Part model, mm, in its own coordinate system. A direction names the side the tool comes from. Round coordinates to 2 decimals unless told otherwise and drop trailing zeros. Loops run counter-clockwise (first coordinate to the right, second up) from the corner with the lowest first, then second, coordinate; pieces in that order, holes last.
1) Probe line 1 (Y direction, x = -3.81, z = -8.5); line 2 (X direction, y = 5.5, z = -10.5); line 3 (Y direction, x = -0.75, z = -4). List the from-to ranges inside material, lowest first.
2) Band-saw the part on C-C, the plane x = -17.75. Write the cut outline in (y, z).
3) Band-saw the part on B-B, the plane y = 10. Write the cut outline in (x, z), then the cut area to 3 significant figures.
4) Drop flat-ended pins along their axis: P1, Ø4, axis at x = -3.5, y = 11, coming from the +Z side; P2, Ø2, axis at y = 4, z = -7, coming from the -X side; P3, Ø3, axis at y = 10.5, z = -4.5, coming from the +X side; P4, Ø4, axis at y = 8, z = -7, coming from the -X side. Give the stop position or say it passes through.
5) 3-axis set-ups, long thin cutter, end or side, ignore diameter. For faces 1 (the flat face through (-4, 6, -4.826)), 2 (the cylindrical face through (-6.474, 11.614, -8.082)): which of +Z, -Z, +X, -X, +Y, -Y reach the whole face in a straight line?
6) Mould opens along X. For faces 3 (the cylindrical face through (-4.05, 10.73, -8.08)), 4 (the flat face through (-7.62, 7, -8)), 5 (the flat face through (-4, 6, -11.43)) say: +X half, -X half, draft (parallel to the pull), parting line (faces both ways), or undercut.
7) Band-saw the part on D-D, the plane y = 12.25. Write the cut outline in (x, z).
8) Band-saw the part on A-A, the plane x = -3. Write the cut outline in (y, z).
Autodesk Inventor part; units mm, degrees
ref_plane "YZ Plane" through (0, 0, 0) normal (1, 0, 0) x (0, 1, 0)
ref_plane "XZ Plane" through (0, 0, 0) normal (0, 1, 0) x (-1, 0, 0)
ref_plane "XY Plane" through (0, 0, 0) normal (0, 0, 1) x (1, 0, 0)
sketch "Sketch1" plane through (0, 0, 0) normal (0, 1, 0) x (-1, 0, 0)
  line L0 (0, 0) -> (21.59, 0)
  line L1 (21.59, 0) -> (21.59, -22.86)
  line L2 (21.59, -22.86) -> (0, -22.86)
  line L3 (0, -22.86) -> (0, 0)
  line L4 (6.35, 0) -> (6.35, -22.86) construction
  circle A0 centre (8.382, -3.7846) radius 0.762
  circle A1 centre (8.382, -19.0754) radius 0.762
  line L5 (6.35, -3.7846) -> (7.62, -3.7846) construction
  line L6 (8.382, -3.0226) -> (8.382, 0) construction
  line L7 (7.62, -19.0754) -> (6.35, -19.0754) construction
  line L8 (8.382, -19.8374) -> (8.382, -22.86) construction
  line L9 (17.653, -10.287) -> (15.367, -10.287) construction
  line L10 (15.367, -10.287) -> (15.367, -12.573) construction
  line L11 (15.367, -12.573) -> (17.653, -12.573) construction
  line L12 (17.653, -12.573) -> (17.653, -10.287) construction
  line L13 (17.653, -11.43) -> (15.367, -11.43) construction
  line L14 (16.51, -10.287) -> (16.51, -12.573) construction
  line L15 (8.382, -19.0754) -> (8.382, -3.7846) construction
  point P0 (6.35, -11.43)
  dimension "d0" = 22.86
  dimension "d1" = 21.59
  dimension "d2" = 1.524
  dimension "d3" = 1.524
  dimension "d4" = 1.27
  dimension "d6" = 1.27
  dimension "d10" = 15.24
  dimension "d11" = 2.286
  dimension "d12" = 2.286
  dimension "d13" = 10.16
  dimension "d14" = 16.51
  dimension "d30" = 15.2908
  dimension "d31" = 3.0226
extrude "Extrusion1" add sketch "Sketch1" along normal blind 3.81
sketch "Sketch2" plane through (0, 3.81, 0) normal (0, 1, 0) x (1, 0, 0)
  line L0 (-21.59, 22.86) -> (-21.59, 0)
  line L1 (-21.59, 11.43) -> (0, 11.43) construction
  line L2 (0, 0) -> (0, 22.86)
  line L3 (0, 11.43) -> (-7.62, 11.43)
  line L4 (-7.62, 11.43) -> (-7.62, 4.826)
  line L5 (-7.62, 4.826) -> (0, 4.826)
  line L6 (0, 4.826) -> (0, 11.43)
  dimension "d17" = 6.604
  dimension "d18" = 7.62
extrude "Extrusion2" add sketch "Sketch2" along normal blind 8.89
fillet "Fillet1" radius 3.81 2 edges at (-7.62, 12.7, -8.128) (0, 12.7, -8.128)
sketch "Sketch3" plane through (-7.62, 3.81, -4.826) normal (0, 0, 1) x (1, 0, 0)
  arc A0 (7.62, 5.08) -> (0, 5.08) centre (3.81, 5.08) ccw
  circle A1 centre (3.81, 5.08) radius 1.8542
  point P0 (7.62, -3.81)
  dimension "d22" = 3.7084
extrude "Extrusion4" cut sketch "Sketch3" against normal through all
chamfer "Chamfer1" distance 1.27 angle 45 1 edges at (-7.62, 3.81, -8.128)
fillet "Fillet2" radius 1.27 4 edges at (-21.59, 1.905, 0) (0, 1.905, 0) (0, 1.905, -22.86) (-21.59, 1.905, -22.86)
equation "\"d3\" = d2"
equation "\"d6\" = d4"
equation "\"d31\" = -0.5 * d2 + 0.5 * d0 - 0.5 * d30"
properties part number "Mount for TMP007 Sensor"
Reported:
1. line 1: y = 0 to 7.04, 10.74 to 12.7
1. line 2: x = -7.62 to 0
1. line 3: y = 0 to 3.81
2. outline: (0, -22.86) - (3.81, -22.86) - (3.81, 0) - (0, 0) - close
3. outline: (-7.45, -11.43) - (-5.3, -11.43) - (-5.3, -4.83) - (-7.45, -4.83) - close; (-2.32, -11.43) - (-0.17, -11.43) - (-0.17, -4.83) - (-2.32, -4.83) - close
3. area: 28.5 mm2
4. P1: stops at z = -4.83
4. P2: stops at x = -21.59
4. P3: stops at x = 0
4. P4: stops at x = -7.62
5. face 1: +Z, +X, -X, +Y
5. face 2: +Z, -Z, -X, +Y
6. face 3: undercut
6. face 4: -X half
6. face 5: draft
7. outline: (-5.61, -11.43) - (-2.01, -11.43) - (-2.01, -4.83) - (-5.61, -4.83) - close
8. outline: (0, -22.86) - (3.81, -22.86) - (3.81, -11.43) - (7.22, -11.43) - (7.22, -4.83) - (3.81, -4.83) - (3.81, 0) - (0, 0) - close; (10.56, -11.43) - (12.61, -11.43) - (12.61, -4.83) - (10.56, -4.83) - close
